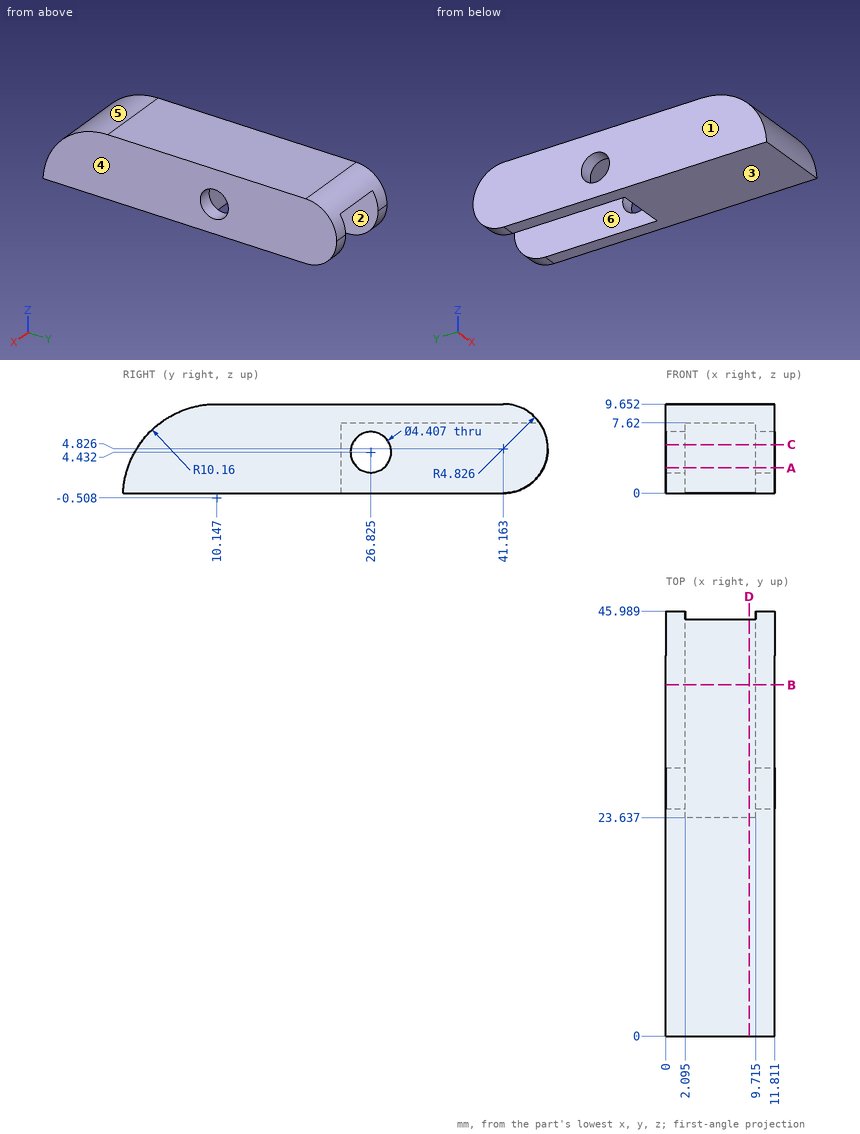
The drawing under review shows one solid part. Ordinate dimensions are in mm from its lowest x, y, z. A direction names the side the tool comes from. Round coordinates to 2 decimals unless told otherwise and drop trailing zeros. Write each loop counter-clockwise with the first axis right and the second up, starting at its lowest first coordinate (ties: lowest second). Pieces come first, ordered by that corner, then holes. Notation, with made-up numbers: (58, 2) - (114, 2) arc R27 cw to (114, 41) - close; hole circle Ø8 at (38, -5). An arc over 180 degrees is marked (long way). Use a Markdown table: item, result. Add a question column.
1. We need section D-D (x = 9). State the section outline as (y, z) points (1 decimal).
2. Mouldability with a two-part tool opening along X and no side actions: class the marked faces 1, 2, 3 and 4 as +X half, -X half, draft (parallel to the pull), parting line (faces both ways), or undercut.
3. We need section B-B (y = 38). State the section outline as (x, z) points (1 decimal).
4. Wall thickness on probe 1 along X at (y, z) = (38, 5.5) (1 decimal); probe 2 along Z at (x, y) = (9.5, 8.5); probe 3 along Z at (x, y) = (2.75, 30.5): over which ranges is each line inside the solid? List them lowest first.
5. Clearance check with flat-ended pins moving along their axes: pin 1 (2.5 mm diameter, centred on x = 5.5, z = 3, fed in from +Y); pin 2 (1 mm diameter, centred on x = 6, z = 6.5, fed in from -Y) (1 decimal); pin 3 (5 mm diameter, centred on y = 13.5, z = 1.5, fed in from -X); pin 4 (1 mm diameter, centred on x = 2.5, z = 7.5, fed in from +Y). State where each tip first meets the part, or that it passes through.
6. We need section A-A (z = 2.75). State the section outline as (x, y) points (1 decimal).
7. We need section C-C (z = 5.25). State the section outline as (x, y) points (1 decimal).
8. For the marked faces 5 and 6, list the 3-axis set-ups (+Z, -Z, +X, -X, +Y, -Y) from which the entire face can be reached by the end or side of a thin tool; tool diameter is ignored.
Output:
| question | item | result |
|---|---|---|
| 1 | outline | (0, 0) - (23.6, 0) - (23.6, 7.6) - (45.1, 7.6) arc R4.8 ccw to (41.2, 9.7) - (10.1, 9.7) arc R10.2 ccw to start |
| 2 | face 1 | -X half |
| 2 | face 2 | undercut |
| 2 | face 3 | draft |
| 2 | face 4 | +X half |
| 3 | outline | (0, 0) - (2.1, 0) - (2.1, 7.6) - (9.7, 7.6) - (9.7, 0) - (11.8, 0) - (11.8, 9.7) - (0, 9.7) - close |
| 4 | probe 1 | x = 0 to 2.1, 9.7 to 11.8 |
| 4 | probe 2 | z = 0 to 9.52 |
| 4 | probe 3 | z = 7.62 to 9.65 |
| 5 | pin 1 | stops at y = 23.64 |
| 5 | pin 2 | stops at y = 2.3 |
| 5 | pin 3 | stops at x = 0 |
| 5 | pin 4 | stops at y = 45.36 |
| 6 | outline | (0, 0.5) - (11.8, 0.5) - (11.8, 25.4) - (9.7, 25.4) - (9.7, 23.6) - (2.1, 23.6) - (2.1, 25.4) - (0, 25.4) - close; (0, 28.2) - (2.1, 28.2) - (2.1, 45.5) - (0, 45.5) - close; (9.7, 28.2) - (11.8, 28.2) - (11.8, 45.5) - (9.7, 45.5) - close |
| 7 | outline | (0, 1.8) - (11.8, 1.8) - (11.8, 24.8) - (9.7, 24.8) - (9.7, 23.6) - (2.1, 23.6) - (2.1, 24.8) - (0, 24.8) - close; (0, 28.9) - (2.1, 28.9) - (2.1, 46) - (0, 46) - close; (9.7, 28.9) - (11.8, 28.9) - (11.8, 46) - (9.7, 46) - close |
| 8 | face 5 | +Z, +X, -X, -Y |
| 8 | face 6 | -Z, +Y |
